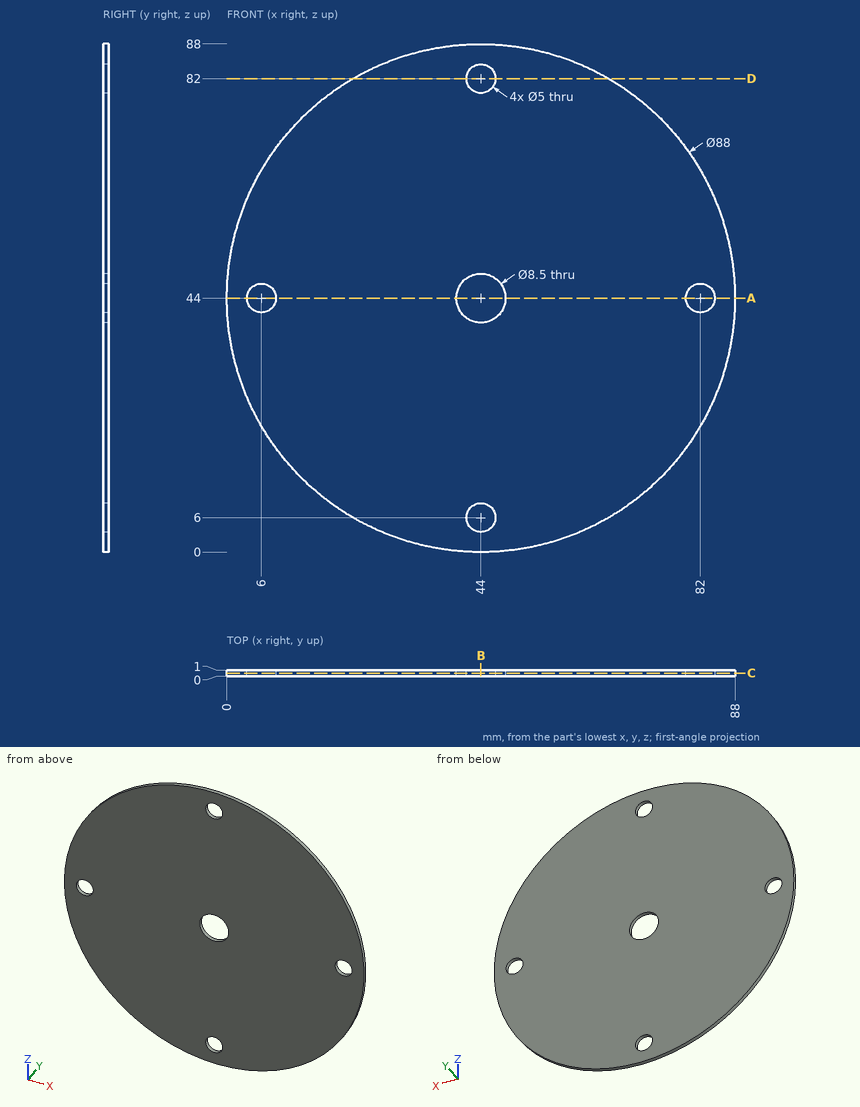
For this review, use the dimensioned drawing (mm, ordinates from the lowest corner) and the shaded views. Coordinates: 2 decimals unless noted, no trailing zeros. Loops run counter-clockwise (first coordinate to the right, second up) from the corner with the lowest first, then second, coordinate; pieces in that order, holes last. Notation, with made-up numbers: (8, 43) -> (57, 43) arc R16 ccw to (57, 49) -> close; hole circle Ø3 at (89.25, 77.5). An arc over 180 degrees is marked (long way). Return JSON: item names as keys, results as strings. Group by question number.
(1) Consider section A-A, the plane z = 44. Give the boundary of the cut face in (x, y).
(2) Consider section C-C, the plane y = 0.5. Give the boundary of the cut face in (x, z).
(3) For pin 1 Ø4.5 at (x, z) = (44, 6) entering from -Y, flat-tipped, find the tip position at first contact; note if it passes through.
(4) To check wall thickness, follow L1, parallel to Z at x = 44, y = 0.6; L2, parallel to Z at x = 82, y = 0.6; L3, parallel to Z at x = 26, y = 0.95. State the ranges of each line that lie inside material, in increasing order.
(5) Consider section D-D, the plane z = 82. Give the boundary of the cut face in (x, y).
(6) Consider section B-B, the plane x = 44. Give the boundary of the cut face in (y, z).
Results below:
{
 "1": {"outline": "(0, 0) -> (3.5, 0) -> (3.5, 1) -> (0, 1) -> close; (8.5, 0) -> (39.75, 0) -> (39.75, 1) -> (8.5, 1) -> close; (48.25, 0) -> (79.5, 0) -> (79.5, 1) -> (48.25, 1) -> close; (84.5, 0) -> (88, 0) -> (88, 1) -> (84.5, 1) -> close"},
 "2": {"outline": "circle Ø88 at (44, 44); hole circle Ø5 at (6, 44); hole circle Ø8.5 at (44, 44); hole circle Ø5 at (44, 6); hole circle Ø5 at (44, 82); hole circle Ø5 at (82, 44)"},
 "3": {"pin 1": "passes through"},
 "4": {"L1": "z = 0 to 3.5, 8.5 to 39.75, 48.25 to 79.5, 84.5 to 88", "L2": "z = 21.82 to 41.5, 46.5 to 66.18", "L3": "z = 3.85 to 84.15"},
 "5": {"outline": "(21.82, 0) -> (41.5, 0) -> (41.5, 1) -> (21.82, 1) -> close; (46.5, 0) -> (66.18, 0) -> (66.18, 1) -> (46.5, 1) -> close"},
 "6": {"outline": "(0, 0) -> (1, 0) -> (1, 3.5) -> (0, 3.5) -> close; (0, 8.5) -> (1, 8.5) -> (1, 39.75) -> (0, 39.75) -> close; (0, 48.25) -> (1, 48.25) -> (1, 79.5) -> (0, 79.5) -> close; (0, 84.5) -> (1, 84.5) -> (1, 88) -> (0, 88) -> close"}
}
